```python
from build123d import *

# Parameters (mm, degrees)
SOCKET_OUTER_EYE_AND_MOUTHS_START = -2.2
SKETCH1_R                         = 3.5
SKETCH1_R_2                       = 2.2
SOCKET_OUTER_EYE_AND_MOUTHS_DEPTH = 4.4
ROD_CONNECTION_NECK_START         = -2
SKETCH2_W                         = 4
SKETCH2_H                         = 5.3
ROD_CONNECTION_NECK_DEPTH         = 4
SKETCH3_R                         = 1.05
D2P1_ROD_BOND_BORE_DEPTH          = 2.7


# Read off the part's stored shape, not the designer's step: Spherical_Socket_D5p05
with BuildPart() as part:
    # Sketch1 → Socket_Outer_Eye_And_Mouths (new body)
    with BuildSketch(Plane.XY.offset(SOCKET_OUTER_EYE_AND_MOUTHS_START)):
        Circle(SKETCH1_R)
        Circle(SKETCH1_R_2, mode=Mode.SUBTRACT)
    extrude(amount=SOCKET_OUTER_EYE_AND_MOUTHS_DEPTH)

    # Sketch2 → Rod_Connection_Neck (add)
    with BuildSketch(Plane.XY.offset(ROD_CONNECTION_NECK_START)):
        with Locations((0, -4.85)):
            Rectangle(SKETCH2_W, SKETCH2_H)
    extrude(amount=ROD_CONNECTION_NECK_DEPTH)

    # Spherical_Socket_D5p05 outline → Spherical_Socket_D5p05 (revolve, cut)
    with BuildSketch(Plane.XZ):
        with BuildLine():
            Line((2.199999999, 1.239203375), (2.199999999, -1.239203375))
            ThreePointArc((2.199999999, -1.239203375), (2.525, 0), (2.199999999, 1.239203375))
        make_face()
    revolve(axis=Axis((0, 0, 0), (0, 0, 1)), mode=Mode.SUBTRACT)

    # Sketch3 → D2p1_Rod_Bond_Bore (cut)
    with BuildSketch(Plane.XZ.offset(7.5)):
        with Locations(Location((0, 0, 0), (0, 0, 270))):
            Circle(SKETCH3_R)
    extrude(amount=-D2P1_ROD_BOND_BORE_DEPTH, mode=Mode.SUBTRACT)


solid = part.part
```
Source: CAD feature listing. Evaluate the final solid. Frame: model axes, mm. A direction names the side the tool comes from. Coordinates: 2 decimals unless noted, no trailing zeros. Loops run counter-clockwise (first coordinate to the right, second up) from the corner with the lowest first, then second, coordinate; pieces in that order, holes last. Notation, with made-up numbers: M 36,-14.5 L 67,-14.5 A21 ccw 67,17.5 Z; hole C -12.75,-11 d9. An arc over 180 degrees is marked long. Put each result on its own line as item: value. Start each with the question number.
1) Cut plane B-B on z = 0. Return the cut outline in (x, y) (3 decimals), then the cut area to 3 significant figures.
2) Reachability of faces 5 (the face through (2.1, 0.66, -1.73)), 6 (the face through (-2, -5, 0)), 7 (the face through (2, -5, 0)) from +Z, -Z, +X, -X, +Y, -Y: full face, straight path, thin tool, end or side. Return the list, or none.
3) Cut plane D-D on z = -1.45. Return the cut outline in (x, y), then the cut area to 3 significant figures.
4) Contact query for flat-ended pins moving along their axis: pin 1 Ø0.6 at (x, z) = (-0.5, -0.5) entering from -Y; pin 2 Ø1.2 at (y, z) = (-5, 1) entering from +X; pin 3 Ø3.5 at (x, y) = (0, 0) entering from -Z; pin 4 Ø2 at (y, z) = (-4, 0) entering from -X. Output: stop coordinate, or through.
5) Cut plane C-C on y = 0. Return the cut outline in (x, z) (3 decimals), then the cut area to 3 significant figures.
6) Cut plane A-A on x = 0. Return the cut outline in (y, z) (3 decimals).
7) Pull-direction query (Z, two-part tool) for faces 1 (the face through (0, -4.8, 0)), 2 (the face through (0.32, -6.17, -1)), 3 (the face through (-1, -7.5, 1)), 4 (the face through (-2, -2, 2.2)); classes: pulls with the +Z half, pulls with the -Z half, needs draft (parallel to the pull), parting line crosses it, or undercut.
8) Ray query, L1, parallel to Y at x = 0, z = 1.95; L2, parallel to X at y = -7, z = 0; L3, parallel to Z at x = -2, y = -1.25. Return the intervals inside material, ascending. Write a range as from..to.
The answers:
1. outline: M -2,-7.5 L -1.05,-7.5 L -1.05,-4.8 L 1.05,-4.8 L 1.05,-7.5 L 2,-7.5 L 2,-2.872 A3.5 ccw long -2,-2.872 Z; hole C 0,0 d5.05
1. area: 29.6 mm²
2. face 5: +Z, -Z
2. face 6: +Z, -Z, -X, -Y
2. face 7: +Z, -Z, +X, -Y
3. outline: M -2,-7.5 L 2,-7.5 L 2,-2.87 A3.5 ccw long -2,-2.87 Z; hole C 0,0 d4.4
3. area: 40.1 mm²
4. pin 1: stops at y = -4.8
4. pin 2: stops at x = 2
4. pin 3: passes through
4. pin 4: stops at x = -2
5. outline: M -3.5,-2.2 L -2.2,-2.2 L -2.2,-1.239 A2.525 cw -2.2,1.239 L -2.2,2.2 L -3.5,2.2 Z; M 2.2,-2.2 L 3.5,-2.2 L 3.5,2.2 L 2.2,2.2 L 2.2,1.239 A2.525 cw 2.2,-1.239 Z
5. area: 10.4 mm²
6. outline: M -7.5,-2 L -3.5,-2 L -3.5,-2.2 L -2.2,-2.2 L -2.2,-1.239 A2.525 cw -2.2,1.239 L -2.2,2.2 L -3.5,2.2 L -3.5,2 L -7.5,2 L -7.5,1.05 L -4.8,1.05 L -4.8,-1.05 L -7.5,-1.05 Z; M 2.2,-2.2 L 3.5,-2.2 L 3.5,2.2 L 2.2,2.2 L 2.2,1.239 A2.525 cw 2.2,-1.239 Z
7. face 1: undercut
7. face 2: undercut
7. face 3: needs draft
7. face 4: pulls with the +Z half
8. L1: y = -7.5..-2.2, 2.2..3.5
8. L2: x = -2..-1.05, 1.05..2
8. L3: z = -2.2..-0.9, 0.9..2.2
